Model file for the job. Use its own axes, mm. Face numbers are marked on the shaded views. A direction names the side the tool comes from. Round coordinates to 2 decimals unless told otherwise and drop trailing zeros. Loops run counter-clockwise (first coordinate to the right, second up) from the corner with the lowest first, then second, coordinate; pieces in that order, holes last.
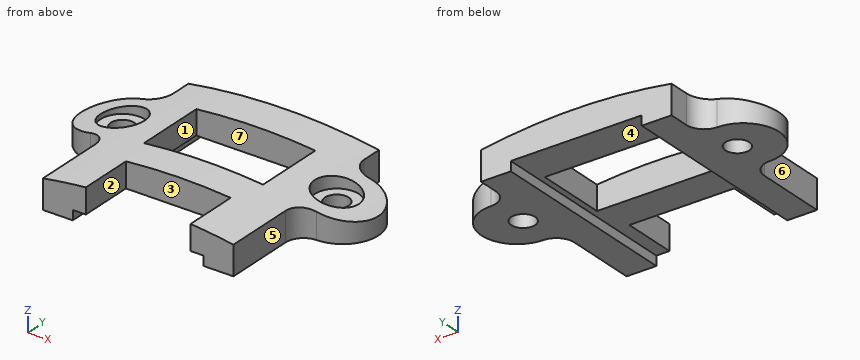
from build123d import *

# Parameters (mm, degrees)
MAIN_DEPTH               = 5.1
SKETCH1_W                = 10
SKETCH1_H                = 6
SENSOR_CUT_DEPTH         = 5.1
MOUNTING_EARS_DEPTH      = 3
SKETCH4_R                = 1
MOUNT_HOLES_DEPTH        = 3
SKETCH9_R                = 1.85
CUT_EXTRUDE1_DEPTH       = 1.5
CIRCULAR_FRONT_CUT_REACH = 23.474
SKETCH6_W                = 11
SKETCH6_H                = 16.7
PCB_CUT_DEPTH            = 0.8
FILLET3_R                = 1.5


with BuildPart() as part:
    # Sketch2 → main (new body)
    with BuildSketch(Plane.XY):
        Polygon((-4.4, -8.35), (-8, -8.35), (-8, 8.35), (8, 8.35), (8, -8.35), (4.4, -8.35), (4.4, -3.75), (-4.4, -3.75), align=None)
    extrude(amount=MAIN_DEPTH)

    # Sketch1 → sensor_cut (cut)
    with BuildSketch(Plane.XY):
        with Locations((0, 2.15)):
            Rectangle(SKETCH1_W, SKETCH1_H)
    extrude(amount=SENSOR_CUT_DEPTH, mode=Mode.SUBTRACT)

    # Sketch3 → mounting_ears (add)
    with BuildSketch(Plane(origin=(0, 0, 0), x_dir=(-1, 0, 0), z_dir=(0, 0, -1))):
        with BuildLine():
            Line((9.5, -0.85), (8, -0.85))
            Line((8, -0.85), (8, 5.15))
            Line((8, 5.15), (9.5, 5.15))
            ThreePointArc((9.5, 5.15), (12.5, 2.15), (9.5, -0.85))
        make_face()
        with BuildLine():
            Line((-8, 5.15), (-9.5, 5.15))
            ThreePointArc((-9.5, 5.15), (-12.5, 2.15), (-9.5, -0.85))
            Line((-9.5, -0.85), (-8, -0.85))
            Line((-8, -0.85), (-8, 5.15))
        make_face()
    extrude(amount=-MOUNTING_EARS_DEPTH)

    # Sketch4 → mount_holes (cut)
    with BuildSketch(Plane.XY.offset(3)):
        with Locations((-9, 2.15)):
            Circle(SKETCH4_R)
    mount_holes = extrude(amount=-MOUNT_HOLES_DEPTH, mode=Mode.SUBTRACT)

    # Sketch9 → Cut-Extrude1 (cut)
    with BuildSketch(Plane.XY.offset(3)):
        with Locations((-9, 2.15)):
            Circle(SKETCH9_R)
    cut_extrude1 = extrude(amount=-CUT_EXTRUDE1_DEPTH, mode=Mode.SUBTRACT)

    # Mirror1: mount_holes, Cut-Extrude1 across plane
    add(mount_holes.mirror(Plane(origin=(0, 0, 0), x_dir=(0, 0, 1), z_dir=(1, 0, 0))), mode=Mode.SUBTRACT)
    add(cut_extrude1.mirror(Plane(origin=(0, 0, 0), x_dir=(0, 0, 1), z_dir=(1, 0, 0))), mode=Mode.SUBTRACT)

    # circular_front_cut: up to this face of the body (flat: up to its plane)
    circular_front_cut_end = Plane(part.part.faces().sort_by_distance((-6.2, -8.35, 2.55))[0])
    # Sketch5 → circular_front_cut (cut, up to the picked face)
    with BuildSketch(Plane(origin=(0, 8.35, 0), x_dir=(1, 0, 0), z_dir=(0, 1, 0)), mode=Mode.PRIVATE) as circular_front_cut_sk1:
        with BuildLine():
            Line((-12.5, -1.5), (-12.5, -9.92320486))
            Line((-12.5, -9.92320486), (12.5, -9.92320486))
            Line((12.5, -9.92320486), (12.5, -1.5))
            ThreePointArc((12.5, -1.5), (0, -3.087708172), (-12.5, -1.5))
        make_face()
    circular_front_cut_tool1 = split(extrude(circular_front_cut_sk1.sketch, amount=-CIRCULAR_FRONT_CUT_REACH, mode=Mode.PRIVATE), bisect_by=circular_front_cut_end, keep=Keep.BOTH, mode=Mode.PRIVATE)
    add(circular_front_cut_tool1.solids().sort_by(Axis((0, 8.35, 6.227394), (0, -1, 0)))[0], mode=Mode.SUBTRACT)

    # Sketch6 → pcb_cut (cut)
    with BuildSketch(Plane(origin=(0, 0, 0), x_dir=(-1, 0, 0), z_dir=(0, 0, -1))):
        Rectangle(SKETCH6_W, SKETCH6_H)
    extrude(amount=-PCB_CUT_DEPTH, mode=Mode.SUBTRACT)

    # Fillet3
    fillet3_edges = [part.edges().sort_by_distance(p)[0] for p in [
        (-8, -0.85, 1.221779445),
        (-8, 5.15, 1.221779445),
        (8, 5.15, 1.221779445),
        (8, -0.85, 1.221779445),
    ]]
    fillet(fillet3_edges, radius=FILLET3_R - 0.0001)  # a hair under: the kernel refuses the full size


solid = part.part
Q1. Tool access for the marked faces 4, 5, 6 and 7: list every direction of +Z, -Z, +X, -X, +Y, -Y with a clear straight run to the whole face (end or side of a thin tool).
Q2. Slice it at D-D on x = -9. Give the cut face in (y, z).
Q3. Slice it at C-C on y = 0. Give the cut face in (x, z), plus the area to 3 significant figures.
Q4. Slice it at B-B on x = -1.5. Give the cut face in (y, z), plus the area to 3 significant figures.
Q5. Pull direction Y, two halves, no side cores. Call the marked faces 1, 2 and 3: pulls with the +Y half, pulls with the -Y half, needs draft (parallel to the pull), parting line crosses it, or undercut.
Q6. Flat gauge pins, fed straight in: P1, Ø1.1, axis at x = -2.5, z = 2, coming from the -Y side; P2, Ø6, axis at x = 9, y = 2.15, coming from the +Z side; P3, Ø0.6, axis at y = 2.5, z = 1.5, coming from the +X side; P4, Ø4, axis at x = 9, y = 2, coming from the +Z side. Where does each tip first touch, or does it go through?
Q7. Probe line 1 (X direction, y = -4, z = 1.4); line 2 (Y direction, x = 4.25, z = 2.2); line 3 (X direction, y = -6, z = 0.5). List the from-to ranges inside material, lowest first.
Q8. Slice it at A-A on y = 2.15. Give the cut face in (x, z).
Reply:
1. face 4: -Z, +Y, -Y
1. face 5: +Z, -Z, +X, -Y
1. face 6: +Z, -Z, -X, -Y
1. face 7: +Z, -Z
2. outline: (-0.94, 0) - (1.15, 0) - (1.15, 1.5) - (0.3, 1.5) - (0.3, 2.27) - (-0.94, 2.27) - close; (3.15, 0) - (5.24, 0) - (5.24, 2.27) - (4, 2.27) - (4, 1.5) - (3.15, 1.5) - close
3. outline: (-11.59, 0) - (-5.5, 0) - (-5.5, 0.8) - (-5, 0.8) - (-5, 2.84) arc R50 ccw to (-11.59, 1.73) - close; (5, 0.8) - (5.5, 0.8) - (5.5, 0) - (11.59, 0) - (11.59, 1.73) arc R50 ccw to (5, 2.84) - close
3. area: 30.3 mm2
4. outline: (-3.75, 0.8) - (-0.85, 0.8) - (-0.85, 3.07) - (-3.75, 3.07) - close; (5.15, 0.8) - (8.35, 0.8) - (8.35, 3.07) - (5.15, 3.07) - close
4. area: 13.8 mm2
5. face 1: undercut
5. face 2: needs draft
5. face 3: pulls with the -Y half
6. P1: stops at y = -3.75
6. P2: stops at z = 2.73
6. P3: stops at x = 12.5
6. P4: stops at z = 2.6
7. line 1: x = -8 to -4.4, 4.4 to 8
7. line 2: y = -3.75 to -0.85, 5.15 to 8.35
7. line 3: x = -8 to -5.5, 5.5 to 8
8. outline: (-12.5, 0) - (-10, 0) - (-10, 1.5) - (-10.85, 1.5) - (-10.85, 1.9) arc R50 ccw to (-12.5, 1.5) - close; (-8, 0) - (-5.5, 0) - (-5.5, 0.8) - (-5, 0.8) - (-5, 2.84) arc R50 ccw to (-7.15, 2.57) - (-7.15, 1.5) - (-8, 1.5) - close; (5, 0.8) - (5.5, 0.8) - (5.5, 0) - (8, 0) - (8, 1.5) - (7.15, 1.5) - (7.15, 2.57) arc R50 ccw to (5, 2.84) - close; (10, 0) - (12.5, 0) - (12.5, 1.5) arc R50 ccw to (10.85, 1.9) - (10.85, 1.5) - (10, 1.5) - close
